```python
from build123d import *

# Parameters (mm, degrees)
F2_T = -2.5
F3_R = 5


with BuildPart() as f1:
    # F0 (on Front) → F1 (revolve)
    with BuildSketch(Plane.XZ):
        Polygon((20.32, 15.2080524429), (20.32, 51.7584940429), (0, 51.7584940429), (0, -189.1371041323), (17.78, -189.1371041323), (17.78, 10.8628958677), align=None)
    revolve(axis=Axis((0, 0, -68.6893050447), (0, 0, -1)))

    # F2
    f2_openings = [f1.faces().sort_by_distance(p)[0] for p in [
        (0, 0, 51.758494),
        (0, 0, -189.137104),
    ]]
    offset(amount=F2_T, openings=f2_openings, kind=Kind.INTERSECTION)

    # F3
    f3_edges = [f1.edges().sort_by_distance(p)[0] for p in [
        (-17.78, 0, 10.862896),
        (-20.32, 0, 15.208052),
        (19.05, 0, 13.035474),
    ]]
    fillet(f3_edges, radius=F3_R)


solid = f1.part
```
Check sheet for the modelled part. Datum: model origin and axes. Units: mm. Give positions to 0.01 mm unless a question says otherwise; leave off trailing zeros. Order: outer loops, then holes, each group sorted by start corner. A loop starts at its lowest first (then second) coordinate and runs counter-clockwise, first axis right, second up. Notation, with made-up numbers: M -13.75,75.5 L 0.25,75.5 A8 cw 0.25,87.5 Z; hole C 0.5,-11 d7. An arc over 180 degrees is marked long. Answer in a Markdown table with one row per item.
1) Thickness scan on L1, parallel to Y at x = 0, z = -95.5; L2, parallel to Y at x = 0, z = 39.5; L3, parallel to X at y = -1, z = -43.5. Record the ranges inside material, lowest first. Write a range as [from, to].
Filled sheet:
| item | result |
|---|---|
| L1 | y = [-17.78, -15.28], [15.28, 17.78] |
| L2 | y = [-20.32, -17.82], [17.82, 20.32] |
| L3 | x = [-17.75, -15.25], [15.25, 17.75] |
2) Gauge pin test, flat ends, axial feed: P1, Ø12, axis at y = 11.5, z = -8.5, coming from the -X side; P2, Ø12, axis at y = -15, z = -70.5, coming from the +X side; P3, Ø2, axis at y = -3.5, z = -157.5, coming from the -X side. Record the tip position at first contact, or that the pin passes through.
Filled sheet:
| item | result |
|---|---|
| P1 | stops at x = -16.91 |
| P2 | stops at x = 15.33 |
| P3 | stops at x = -17.6 |
3) Release check for a two-part mould opening along Y. For faces 1 (the conical face through (14.726, -4.637, 11.812)), 2 (the flat face through (0, 18, 51.758)), 3 (the cylindrical face through (-3.85, 17.36, -88.42)), 4 (the cylindrical face through (16.46, 6.83, 34.07)) record: +Y half, -Y half, draft (parallel to the pull), parting line (faces both ways), or undercut.
Filled sheet:
| item | result |
|---|---|
| face 1 | undercut |
| face 2 | draft |
| face 3 | parting line |
| face 4 | undercut |
4) Cross-section at A-A, the plane z = -119. Enter the section's corners in (x, y).
Filled sheet:
| item | result |
|---|---|
| outline | C 0,0 d35.56; hole C 0,0 d30.56 |
